from build123d import *

# Parameters (mm, degrees)
SKETCH2_R               = 1.455
BOSS_EXTRUDE3_DEPTH     = 6
SKETCH3_R               = 2.5
BOSS_EXTRUDE4_DEPTH     = 3
CUT_EXTRUDE1_DEPTH      = 10.669539803
CUT_EXTRUDE1_DEPTH_BACK = 10.669539803
SKETCH4_R               = 0.5
SKETCH6_R               = 1.575
BOSS_EXTRUDE5_DEPTH     = 0.15


with BuildPart() as part:
    # Sketch2 → Boss-Extrude3 (new body)
    with BuildSketch(Plane(origin=(0, 0, 0), x_dir=(0, 0, -1), z_dir=(1, 0, 0))):
        Circle(SKETCH2_R)
    extrude(amount=BOSS_EXTRUDE3_DEPTH)

    # Sketch3 → Boss-Extrude4 (add)
    with BuildSketch(Plane(origin=(6, 0, 0), x_dir=(0, 0, -1), z_dir=(1, 0, 0))):
        Circle(SKETCH3_R)
    extrude(amount=BOSS_EXTRUDE4_DEPTH)

    # Sketch4 → Cut-Extrude1 (cut, two sides: drawn at the far end of the back side and taken through both)
    with BuildSketch(Plane(origin=(0, 0, 0), x_dir=(1, 0, 0), z_dir=(0, 1, 0)).offset(-CUT_EXTRUDE1_DEPTH_BACK)):
        with Locations(Location((3, 0, 0), (0, 0, 270))):
            Circle(SKETCH4_R)
    extrude(amount=CUT_EXTRUDE1_DEPTH + CUT_EXTRUDE1_DEPTH_BACK, mode=Mode.SUBTRACT)

    # Sketch6 → Boss-Extrude5 (add)
    with BuildSketch(Plane.ZY.offset(-3)):
        Circle(SKETCH6_R)
    extrude(amount=BOSS_EXTRUDE5_DEPTH)

    # Sketch7 → Revolve1 (revolve)
    with BuildSketch(Plane.XY, mode=Mode.PRIVATE) as revolve1_sk:
        Polygon((2.85, 1.825), (0, 0.8), (2.85, 0.8), align=None)
    revolve(revolve1_sk.sketch.rotate(Axis((9.45, 0, 0), (-1, 0, 0)), 90), axis=Axis((9.45, 0, 0), (-1, 0, 0)))


solid = part.part
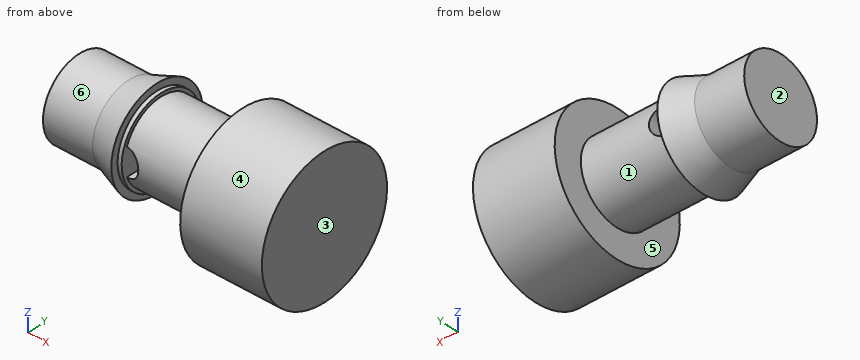
Verification items for the finished model (mm, model axes). Face numbers are marked on the shaded views. A direction names the side the tool comes from. Coordinates: 2 decimals unless noted, no trailing zeros. Loops run counter-clockwise (first coordinate to the right, second up) from the corner with the lowest first, then second, coordinate; pieces in that order, holes last. Notation, with made-up numbers: (74.25, 54) -> (116.25, 54) arc R13 cw to (116.25, 61) -> close; hole circle Ø1 at (60, -37.5). An arc over 180 degrees is marked (long way). Answer as a JSON object with one key per item and string values. Group by question number.
Item 1: Sectioned sample at C-C on x = 4. Record the boundary of the cut face in (y, z) (3 decimals), plus the area to 3 significant figures.
Item 2: Mould release check, pull along X, two halves, no side actions. Record for the marked faces 1, 2, 3 and 4: +X half, -X half, draft (parallel to the pull), parting line (faces both ways), or undercut.
Item 3: Tool access check on the marked faces 5 and 6. Record the directions out of +Z, -Z, +X, -X, +Y, -Y that give a thin tool (end or side, any length) a straight path to the whole face; none if there is none.
Item 4: Scan lines: probe 1 along X at (y, z) = (1.3, -0.8); probe 2 along X at (y, z) = (1.6, -1.25); probe 3 along Y at (x, z) = (1.25, -0.05). Record each from-to range of solid material in increasing order.
Item 5: Sectioned sample at D-D on y = -2. Record the boundary of the cut face in (x, z).
Item 6: Sectioned sample at B-B on y = 0. Record the boundary of the cut face in (x, z) (3 decimals).
Item 7: Depth check by flat-ended pin: pin 1 (1.5 mm diameter, centred on x = 7, z = -2, fed in from -Y); pin 2 (1 mm diameter, centred on x = 7.5, z = 1.5, fed in from -Y); pin 3 (2 mm diameter, centred on x = 2.5, y = -0.5, fed in from -Z) (3 decimals). Enter the tip coordinate at first touch or a pass-through.
Item 8: Sectioned sample at A-A on z = 0. Record the boundary of the cut face in (x, y) (3 decimals), plus the area to 3 significant figures.
Evaluation:
{
 "1": {"outline": "circle Ø2.91 at (0, 0)", "area": "6.65 mm²"},
 "2": {"face 1": "undercut", "face 2": "-X half", "face 3": "+X half", "face 4": "draft"},
 "3": {"face 5": "none", "face 6": "-X"},
 "4": {"probe 1": "x = 2.02 to 3, 6 to 9", "probe 2": "x = 6 to 9", "probe 3": "y = -1.45 to 1.45"},
 "5": {"outline": "(6, -1.5) -> (9, -1.5) -> (9, 1.5) -> (6, 1.5) -> close"},
 "6": {"outline": "(0, -1.455) -> (1.821, -1.455) -> (2.85, -1.825) -> (2.85, -1.575) -> (3, -1.575) -> (3, -1.455) -> (6, -1.455) -> (6, -2.5) -> (9, -2.5) -> (9, 2.5) -> (6, 2.5) -> (6, 1.455) -> (3, 1.455) -> (3, 1.575) -> (2.85, 1.575) -> (2.85, 1.825) -> (1.821, 1.455) -> (0, 1.455) -> close; hole (2.85, -0.477) -> (2.85, 0.477) arc R0.5 ccw to start; hole (3, -0.5) arc R0.5 ccw to (3, 0.5) -> close"},
 "7": {"pin 1": "stops at y = -2.17", "pin 2": "stops at y = -2.29", "pin 3": "stops at z = -1.825"},
 "8": {"outline": "(0, -1.455) -> (1.821, -1.455) -> (2.85, -1.825) -> (2.85, -1.575) -> (3, -1.575) -> (3, 1.575) -> (2.85, 1.575) -> (2.85, 1.825) -> (1.821, 1.455) -> (0, 1.455) -> close; (3.5, -1.455) -> (6, -1.455) -> (6, -2.5) -> (9, -2.5) -> (9, 2.5) -> (6, 2.5) -> (6, 1.455) -> (3.5, 1.455) -> close; hole (2.5, -0.8) -> (2.85, -0.8) -> (2.85, 0.8) -> (2.5, 0.8) -> close", "area": "30.9 mm²"}
}
